The model under review builds one solid part; all positions refer to its coordinate system, in mm. A direction names the side the tool comes from. Round coordinates to 2 decimals unless told otherwise and drop trailing zeros. Order: outer loops, then holes, each group sorted by start corner. A loop starts at its lowest first (then second) coordinate and runs counter-clockwise, first axis right, second up. Notation, with made-up numbers: M 74.5,46 L 86.5,46 A20 cw 86.5,72 Z; hole C -31.5,79 d1. An arc over 180 degrees is marked long. Answer as a JSON object with one key per item and string values. Group by question number.
1) Consider section C-C, the plane z = 326. Write out the cut boundary in (x, y).
2) For faces 5 (the flat face through (280, -291.241, 273)), 6 (the flat face through (107, -179, 600)), 7 (the flat face through (-1, -171.241, 1942)), 8 (the flat face through (252.302, 26, 1942)), 9 (the flat face through (-247.698, 26, 1942)), list the 3-axis set-ups (+Z, -Z, +X, -X, +Y, -Y) from which the entire face can be reached by the end or side of a thin tool; tool diameter is ignored.
3) Consider section A-A, the plane x = 277. Write out the cut boundary in (y, z).
4) Consider section D-D, the plane x = 49.5. Write out the cut boundary in (y, z).
5) Insertion check: pin 1 Ø3 at (y, z) = (-235.5, 844.5) entering from +X; pin 2 Ø1.5 at (x, y) = (152.5, -195.5) entering from -Z. Each pin has a flat end and moves straight along its axis. Give the tip position at first contact, or say it passes through.
6) The part is to be moulded in two halves that separate along Y. For faces 1 (the flat face through (-1, 32, 2500)), 2 (the flat face through (107, 38.759, 854)), 3 (the flat face through (102.302, -84, 277)), 4 (the flat face through (280, -84, 450)), say which applies: +Y half, -Y half, draft (parallel to the pull), parting line (faces both ways), or undercut.
7) Consider section B-B, the plane y = -21. Write out the cut boundary in (x, z), then the cut area to 3 significant figures.
8) To check wall thickness, follow line 1 (Z direction, x = 312, y = -92.5); line 2 (Z direction, x = 160, y = -103); line 3 (Z direction, x = -135, y = -26). State the ranges of each line that lie inside material, in increasing order.
```python
from build123d import *

# Parameters (mm, degrees)
F0_W     = 900
F0_H     = 620
F1_DEPTH = 1400
F2_W     = 682
F2_H     = 500
F3_DEPTH = 430
F4_W     = 500
F4_H     = 400
F5_DEPTH = 1100
F6_W     = 420
F6_H     = 350
F7_DEPTH = 350


with BuildPart() as f1:
    # F0 (on Top) → F1 (new body)
    with BuildSketch(Plane.XY):
        with Locations((2.302444, -81.240896)):
            Rectangle(F0_W, F0_H)
    extrude(amount=F1_DEPTH)

    # F2 (on face) → F3 (cut)
    with BuildSketch(Plane.XZ.offset(391.240896)):
        with Locations((111.302444, 850)):
            Rectangle(F2_W, F2_H)
    extrude(amount=-F3_DEPTH, mode=Mode.SUBTRACT)

    # F4 (on face) → F5 (join)
    with BuildSketch(Plane.XY.offset(1400)):
        with Locations((2.302444, 28.759104)):
            Rectangle(F4_W, F4_H)
    extrude(amount=F5_DEPTH)

    # F6 (on face) → F7 (cut)
    with BuildSketch(Plane.YZ.offset(452.302444)):
        with Locations((-81.240896, 275)):
            Rectangle(F6_W, F6_H)
    extrude(amount=-F7_DEPTH, mode=Mode.SUBTRACT)


solid = f1.part
```
Results list:
{
 "1": {"outline": "M -447.7,-391.24 L 452.3,-391.24 L 452.3,-291.24 L 102.3,-291.24 L 102.3,128.76 L 452.3,128.76 L 452.3,228.76 L -447.7,228.76 Z"},
 "2": {"face 5": "+X", "face 6": "+X, -Y", "face 7": "+Z, +X, -X, -Y", "face 8": "+Z, +X, +Y, -Y", "face 9": "+Z, -X, +Y, -Y"},
 "3": {"outline": "M -391.24,0 L 228.76,0 L 228.76,1400 L -391.24,1400 L -391.24,1100 L 38.76,1100 L 38.76,600 L -391.24,600 Z; hole M -291.24,100 L 128.76,100 L 128.76,450 L -291.24,450 Z"},
 "4": {"outline": "M -391.24,0 L 228.76,0 L 228.76,2500 L -171.24,2500 L -171.24,1400 L -391.24,1400 L -391.24,1100 L 38.76,1100 L 38.76,600 L -391.24,600 Z"},
 "5": {"pin 1": "x = -229.7", "pin 2": "z = 0"},
 "6": {"face 1": "draft", "face 2": "-Y half", "face 3": "undercut", "face 4": "undercut"},
 "7": {"outline": "M -447.7,0 L 452.3,0 L 452.3,100 L 102.3,100 L 102.3,450 L 452.3,450 L 452.3,600 L -229.7,600 L -229.7,1100 L 452.3,1100 L 452.3,1400 L 252.3,1400 L 252.3,2500 L -247.7,2500 L -247.7,1400 L -447.7,1400 Z", "area": "1,350,000 mm^2"},
 "8": {"line 1": "0 to 100, 450 to 600, 1100 to 1400", "line 2": "0 to 100, 450 to 600, 1100 to 2500", "line 3": "0 to 600, 1100 to 2500"}
}
